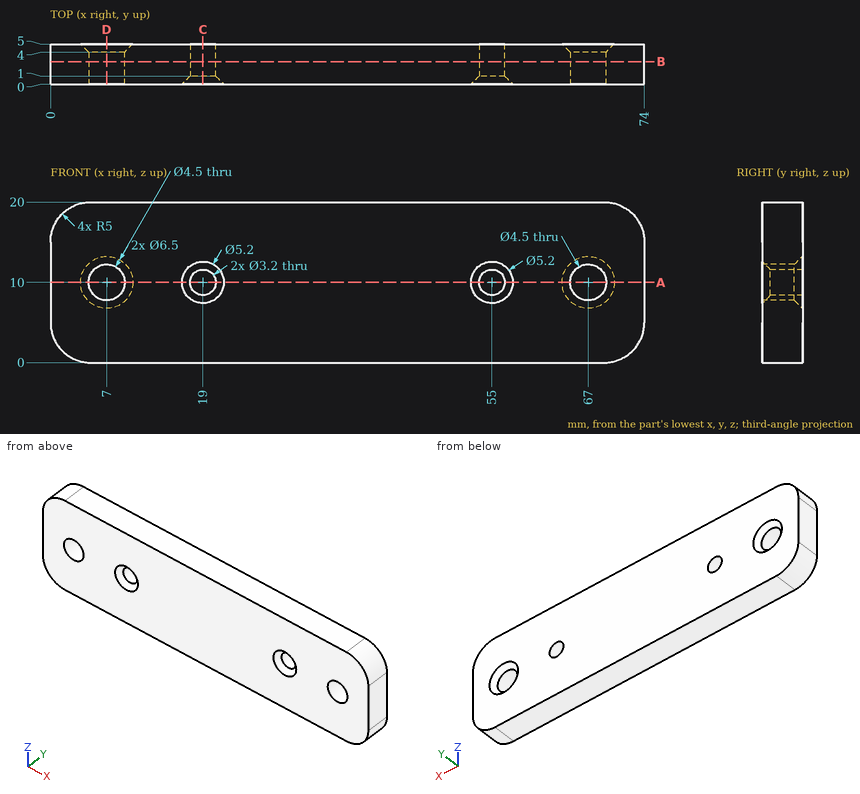
Source: three-view drawing plus pictorial views. Frame: mm from the lowest corner of the part. Round coordinates to 2 decimals unless told otherwise and drop trailing zeros. Write each loop counter-clockwise with the first axis right and the second up, starting at its lowest first coordinate (ties: lowest second). Pieces come first, ordered by that corner, then holes. Notation, with made-up numbers: M 74.5,53.25 L 89.5,53.25 A18 ccw 89.5,81.25 Z; hole C -6,-28 d9. An arc over 180 degrees is marked long. Write item = value, one per line.
Item 1: Material intervals for line 1 along X through (y, z) = (1.1, 10); line 2 along Z through (x, y) = (19, 4.05); line 3 along Z through (x, y) = (7, 3.2), sorted ascending. Write a range as [from, to].
Findings:
line_1 = [0, 4.75], [9.25, 17.4], [20.6, 53.4], [56.6, 64.75], [69.25, 74]
line_2 = [0, 8.4], [11.6, 20]
line_3 = [0, 7.75], [12.25, 20]
Item 2: Section query B-B on y = 2.8. Return loops of the section in (x, z), then the cut area to 3 significant figures.
Findings:
outline = M 0,5 A5 ccw 5,0 L 69,0 A5 ccw 74,5 L 74,15 A5 ccw 69,20 L 5,20 A5 ccw 0,15 Z; hole C 7,10 d4.5; hole C 19,10 d3.2; hole C 55,10 d3.2; hole C 67,10 d4.5
area = 1,410 mm^2
Item 3: Section query C-C on x = 19. Return loops of the section in (y, z), then the cut area to 3 significant figures.
Findings:
outline = M 0,0 L 5,0 L 5,8.4 L 1,8.4 L 0,7.4 Z; M 0,12.6 L 1,11.6 L 5,11.6 L 5,20 L 0,20 Z
area = 83.0 mm^2
Item 4: Section query D-D on x = 7. Return loops of the section in (y, z).
Findings:
outline = M 0,0 L 5,0 L 5,6.75 L 4,7.75 L 0,7.75 Z; M 0,12.25 L 4,12.25 L 5,13.25 L 5,20 L 0,20 Z
Item 5: Pin query (flat end, axial travel): P1, Ø4, axis at x = 55, z = 10, coming from the -Y side; P2, Ø5, axis at x = 67, z = 10, coming from the +Y side. Return the tip coordinate at first contact, or that it passes through.
Findings:
P1 = 0.6
P2 = 4.25
Item 6: Section query A-A on z = 10. Return loops of the section in (x, y).
Findings:
outline = M 0,0 L 4.75,0 L 4.75,4 L 3.75,5 L 0,5 Z; M 9.25,0 L 16.4,0 L 17.4,1 L 17.4,5 L 10.25,5 L 9.25,4 Z; M 20.6,1 L 21.6,0 L 52.4,0 L 53.4,1 L 53.4,5 L 20.6,5 Z; M 56.6,1 L 57.6,0 L 64.75,0 L 64.75,4 L 63.75,5 L 56.6,5 Z; M 69.25,0 L 74,0 L 74,5 L 70.25,5 L 69.25,4 Z
